from build123d import *

# Parameters (mm, degrees)
F0_W     = 304.8
F0_H     = 234.95
F1_DEPTH = 12.7
F3_D     = 16.66748
F5_D     = 10.0838
F6_W     = 12.7
F6_H     = 38.1
F7_DEPTH = 25.4
F8_W     = 38.1
F8_H     = 6.35
F9_DEPTH = 12.7


with BuildPart() as f1:
    # F0 (on Front) → F1 (new body)
    with BuildSketch(Plane.XZ):
        with Locations((152.4, 117.475)):
            Rectangle(F0_W, F0_H)
    extrude(amount=F1_DEPTH)

    # F3 (through all)
    with Locations(Plane.XZ.offset(12.7)):
        with Locations((215.9, 25.4), (88.9, 25.4), (88.9, 209.55), (215.9, 209.55)):
            Hole(F3_D / 2)

    # F5 (through all)
    with Locations(Plane.XZ.offset(12.7)):
        with Locations((263.525, 25.4), (263.525, 209.55), (41.275, 209.55), (41.275, 25.4), (41.275, 117.475), (263.525, 117.475)):
            Hole(F5_D / 2)

    # F6 (on face) → F7 (cut)
    with BuildSketch(Plane.XZ.offset(12.7)):
        with Locations((298.45, 58.7375)):
            Rectangle(F6_W, F6_H)
        with Locations((6.35, 58.7375)):
            Rectangle(F6_W, F6_H)
        with Locations((6.35, 176.2125)):
            Rectangle(F6_W, F6_H)
        with Locations((298.45, 176.2125)):
            Rectangle(F6_W, F6_H)
    extrude(amount=-F7_DEPTH, mode=Mode.SUBTRACT)

    # F8 (on face) → F9 (join)
    with BuildSketch(Plane.XZ.offset(12.7)):
        with Locations((76.2, 238.125)):
            Rectangle(F8_W, F8_H)
        with Locations((228.6, 238.125)):
            Rectangle(F8_W, F8_H)
    extrude(amount=-F9_DEPTH)


solid = f1.part
Here's how the part is built. I have some questions about the finished solid (model axes, mm). A direction names the side the tool comes from. Coordinates: 2 decimals unless noted, no trailing zeros. Order: outer loops, then holes, each group sorted by start corner. A loop starts at its lowest first (then second) coordinate and runs counter-clockwise, first axis right, second up. Notation, with made-up numbers: M -10.75,10 L 18.25,10 A12 ccw 18.25,14 Z; hole C -12,-31.5 d5. An arc over 180 degrees is marked long. Answer as CSV lines item,"result". Start each with the question number.
1. I want a section at A-A, the plane z = 25.4. Write out the boundary of the cut face in (x, y), and give its area (3 significant figures).
2. I want a section at D-D, the plane y = -5.5. Count the separate pieces of the cut face and the enclosed holes in it, and give its area (3 significant figures).
3. I want a section at B-B, the plane x = 215.9. Write out the boundary of the cut face in (y, z).
4. On a 3-axis mill with a long thin cutter (end or side, diameter ignored), from which of +Z, -Z, +X, -X, +Y, -Y can I reach the whole of each face in a straight line? I mean faces 1 (the flat face through (304.8, -6, 215)), 2 (the flat face through (209.55, -6, 238)), 3 (the flat face through (6, -6, 77.788)), 4 (the flat face through (298, -6, 157.162)), 5 (the flat face through (28, -6, 234.95)). Say none if no direction works.
5. I want a section at C-C, the plane z = 172. Write out the boundary of the cut face in (x, y), and give its area (3 significant figures).
6. I need wall thicknesses on line 1 (X direction, y = -1.5, z = 206); line 2 (X direction, y = -11.25, z = 72.5); line 3 (Z direction, x = 193.5, y = -8.5). Which ranges of each line are inside material? Lowest first, please. Write a range as [from, to].
7. We'd pull the mould along X, two halves only. Please class faces 6 (the flat face through (276, -6, 234.95)), 7 (the flat face through (292.1, -6, 58)), 8 (the cylindrical face through (95.513, -6.261, 20.329)): released by +X, released by -X, zero draft, split by the parting line, or undercut.
8. For pin 1 (6.5 mm diameter, centred on x = 296, y = -8, fed in from +Z); pin 2 (6.5 mm diameter, centred on y = -3.5, z = 66.5, fed in from +X); pin 3 (1.9 mm diameter, centred on y = -6.5, z = 237, fed in from +X), each with a flat end and sliding along its axis, tell me the tip position at first contact or that it passes through.
Recorded:
1,outline,"M 0,-12.7 L 36.23,-12.7 L 36.23,0 L 0,0 Z; M 46.32,-12.7 L 80.57,-12.7 L 80.57,0 L 46.32,0 Z; M 97.23,-12.7 L 207.57,-12.7 L 207.57,0 L 97.23,0 Z; M 224.23,-12.7 L 258.48,-12.7 L 258.48,0 L 224.23,0 Z; M 268.57,-12.7 L 304.8,-12.7 L 304.8,0 L 268.57,0 Z"
1,area,"3,190 mm2"
2,separate pieces,"1"
2,enclosed holes,"10"
2,area,"68,800 mm2"
3,outline,"M -12.7,0 L 0,0 L 0,17.07 L -12.7,17.07 Z; M -12.7,33.73 L 0,33.73 L 0,201.22 L -12.7,201.22 Z; M -12.7,217.88 L 0,217.88 L 0,241.3 L -12.7,241.3 Z"
4,face 1,"+Z, -Z, +X, +Y, -Y"
4,face 2,"+Z, +Y, -Y"
4,face 3,"-X, +Y, -Y"
4,face 4,"+X, +Y, -Y"
4,face 5,"+Z, -X, +Y, -Y"
5,outline,"M 12.7,-12.7 L 292.1,-12.7 L 292.1,0 L 12.7,0 Z"
5,area,"3,550 mm2"
6,line 1,"x = [0, 37.69], [44.86, 81.36], [96.44, 208.36], [223.44, 259.94], [267.11, 304.8]"
6,line 2,"x = [12.7, 292.1]"
6,line 3,"z = [0, 234.95]"
7,face 6,"zero draft"
7,face 7,"released by +X"
7,face 8,"undercut"
8,pin 1,"stops at z = 234.95"
8,pin 2,"stops at x = 292.1"
8,pin 3,"stops at x = 247.65"
